The listing builds one solid part. Answer for the finished solid, in the listing's coordinates (mm). Face numbers are marked on the shaded views. A direction names the side the tool comes from. Round coordinates to 2 decimals unless told otherwise and drop trailing zeros. Loops run counter-clockwise (first coordinate to the right, second up) from the corner with the lowest first, then second, coordinate; pieces in that order, holes last. Notation, with made-up numbers: M 72,14 L 101,14 A18 ccw 101,42 Z; hole C 83.5,22 d7. An arc over 180 degrees is marked long. Answer as a JSON object with one key per item and string values.
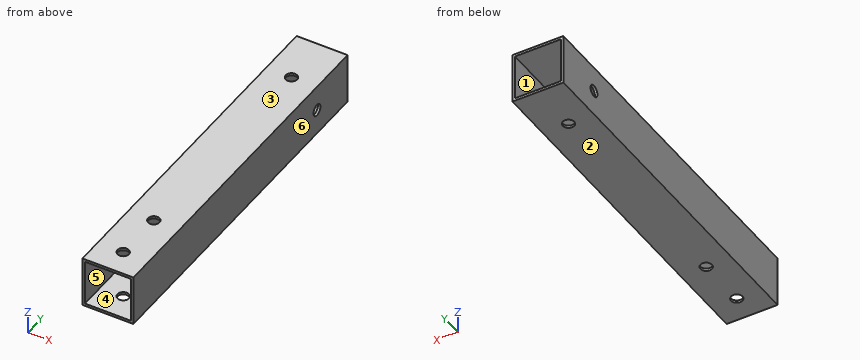
```python
from build123d import *

# Parameters (mm, degrees)
SKETCH1_W           = 20
SKETCH1_H           = 20
SKETCH1_W_2         = 18
SKETCH1_H_2         = 18
BOSS_EXTRUDE1_DEPTH = 140
SKETCH2_R           = 2.25
CUT_EXTRUDE1_DEPTH  = 142.774468788
SKETCH3_R           = 2.25
CUT_EXTRUDE2_DEPTH  = 142.774468788


with BuildPart() as part:
    # Sketch1 → Boss-Extrude1 (new body)
    with BuildSketch(Plane(origin=(0, 0, 0), x_dir=(1, 0, 0), z_dir=(0, 1, 0))):
        Rectangle(SKETCH1_W, SKETCH1_H)
        Rectangle(SKETCH1_W_2, SKETCH1_H_2, mode=Mode.SUBTRACT)
    extrude(amount=BOSS_EXTRUDE1_DEPTH)

    # Sketch2 → Cut-Extrude1 (cut, through all)
    with BuildSketch(Plane.XY.offset(10)):
        with Locations((0, 10)):
            Circle(SKETCH2_R)
        with Locations((0, 30)):
            Circle(SKETCH2_R)
        with Locations((0, 120)):
            Circle(SKETCH2_R)
    extrude(amount=-CUT_EXTRUDE1_DEPTH, mode=Mode.SUBTRACT)

    # Sketch3 → Cut-Extrude2 (cut, through all)
    with BuildSketch(Plane(origin=(10, 0, 0), x_dir=(0, 0, -1), z_dir=(1, 0, 0))):
        with Locations((0, 120)):
            Circle(SKETCH3_R)
    extrude(amount=-CUT_EXTRUDE2_DEPTH, mode=Mode.SUBTRACT)


solid = part.part
```
Item 1: The part is cut by section C-C (z = -6.75). Give the vertices of the cut face in (x, y), then the cut area to 3 significant figures.
Values follow:
{"outline": "M -10,0 L -9,0 L -9,140 L -10,140 Z; M 9,0 L 10,0 L 10,140 L 9,140 Z", "area": "280 mm^2"}
Item 2: Straight lines are drawn through the part: line 1 (Y direction, x = 0, z = -9.35); line 2 (Z direction, x = -1.5, y = 43). For each, find the intervals that lie inside material, in ascending order.
Values follow:
{"line 1": "0 to 7.75, 12.25 to 27.75, 32.25 to 117.75, 122.25 to 140", "line 2": "-10 to -9, 9 to 10"}
Item 3: The part is cut by section A-A (y = 10). Give the vertices of the cut face in (x, z).
Values follow:
{"outline": "M -10,-10 L -2.25,-10 L -2.25,-9 L -9,-9 L -9,9 L -2.25,9 L -2.25,10 L -10,10 Z; M 2.25,-10 L 10,-10 L 10,10 L 2.25,10 L 2.25,9 L 9,9 L 9,-9 L 2.25,-9 Z"}
Item 4: Determine the mould class of the marked faces 3, 4, 5 and 6 for opening direction X: released by +X, released by -X, zero draft, split by the parting line, or undercut.
Values follow:
{"face 3": "zero draft", "face 4": "undercut", "face 5": "undercut", "face 6": "released by +X"}
Item 5: Which of the six approach directions +Z, -Z, +X, -X, +Y, -Y give full straight-line access (tool end or side, diameter ignored) to the marked faces 1 and 2?
Values follow:
{"face 1": "+Y, -Y", "face 2": "-Z, +X, -X, +Y, -Y"}
Item 6: The part is cut by section D-D (y = 120). Give the vertices of the cut face in (x, z), then the cut area to 3 significant figures.
Values follow:
{"outline": "M -10,-10 L -2.25,-10 L -2.25,-9 L -9,-9 L -9,-2.25 L -10,-2.25 Z; M -10,2.25 L -9,2.25 L -9,9 L -2.25,9 L -2.25,10 L -10,10 Z; M 2.25,-10 L 10,-10 L 10,-2.25 L 9,-2.25 L 9,-9 L 2.25,-9 Z; M 2.25,9 L 9,9 L 9,2.25 L 10,2.25 L 10,10 L 2.25,10 Z", "area": "58.0 mm^2"}
Item 7: Flat-ended cylindrical pins translate along their axes: P1, Ø8, axis at x = -6.5, z = -6.5, coming from the -Y side; P2, Ø3.5, axis at x = 0, y = 10, coming from the +Z side. Find the tip coordinate at first contact, or state that the pin passes through.
Values follow:
{"P1": "y = 0", "P2": "through"}
Item 8: The part is cut by section B-B (x = 0). Give the number of separate pieces and of enclosed holes in the cut face, then the cut area to 3 significant figures.
Values follow:
{"separate pieces": "8", "enclosed holes": "0", "area": "253 mm^2"}
